Read the model definition and answer for the solid it produces. Units are mm, in the model's axes. A direction names the side the tool comes from. Coordinates: 2 decimals unless noted, no trailing zeros. Loops run counter-clockwise (first coordinate to the right, second up) from the corner with the lowest first, then second, coordinate; pieces in that order, holes last. Notation, with made-up numbers: (-7.5, 28) - (24.5, 28) arc R15 cw to (24.5, 56) - close; hole circle Ø9 at (29.5, -18). An arc over 180 degrees is marked (long way). Use one line per item in the form item = value.
from build123d import *

# Parameters (mm, degrees)
BOX001_W               = 4
BOX001_H               = 19
BOX001_DEPTH           = 10
BOX001_PLACEMENT_ANGLE = 90
POCKET001_DEPTH        = 5
BOX002_W               = 4
BOX002_H               = 19
BOX002_DEPTH           = 10
POCKET002_DEPTH        = 5
BOX003_W               = 4
BOX003_H               = 19
BOX003_DEPTH           = 10
BOX003_PLACEMENT_ANGLE = -90
POCKET003_DEPTH        = 5
BOX_W                  = 4
BOX_H                  = 19
BOX_DEPTH              = 10
POCKET_DEPTH           = 5
CYLINDER_R             = 3.5
CYLINDER_DEPTH         = 9
CYLINDER001_R          = 5
CYLINDER001_DEPTH      = 12


with BuildPart() as pocket001:
    # Box001 → Box001 (new body)
    with BuildSketch(Plane.XY):
        with Locations((2, 9.5)):
            Rectangle(BOX001_W, BOX001_H)
    extrude(amount=BOX001_DEPTH)


with BuildPart() as pocket001_1:
    # Box001 placement: moved
    add(pocket001.part.moved(Location((-4, -2, 0))).rotate(Axis((-4, -2, 0), (0, 0, 1)), BOX001_PLACEMENT_ANGLE))

    # Sketch001 → Pocket001 (cut)
    with BuildSketch(Plane(origin=(-4, 2, 0), x_dir=(-1, 0, 0), z_dir=(0, 1, 0))):
        Polygon((14.366066, 0), (19, 0), (19, 10), (17.795696, 10), align=None)
    extrude(amount=-POCKET001_DEPTH, mode=Mode.SUBTRACT)


with BuildPart() as pocket002:
    # Box002 → Box002 (new body)
    with BuildSketch(Plane(origin=(2, -4, 0), x_dir=(-1, 0, 0), z_dir=(0, 0, 1))):
        with Locations((2, 9.5)):
            Rectangle(BOX002_W, BOX002_H)
    extrude(amount=BOX002_DEPTH)

    # Sketch002 → Pocket002 (cut)
    with BuildSketch(Plane(origin=(-2, -4, 0), x_dir=(0, -1, 0), z_dir=(-1, 0, 0))):
        Polygon((14.366066, 0), (19, 0), (19, 10), (17.795696, 10), align=None)
    extrude(amount=-POCKET002_DEPTH, mode=Mode.SUBTRACT)


with BuildPart() as pocket003:
    # Box003 → Box003 (new body)
    with BuildSketch(Plane.XY):
        with Locations((2, 9.5)):
            Rectangle(BOX003_W, BOX003_H)
    extrude(amount=BOX003_DEPTH)


with BuildPart() as pocket003_1:
    # Box003 placement: moved
    add(pocket003.part.moved(Location((4, 2, 0))).rotate(Axis((4, 2, 0), (0, 0, 1)), BOX003_PLACEMENT_ANGLE))

    # Sketch003 → Pocket003 (cut)
    with BuildSketch(Plane(origin=(4, -2, 0), x_dir=(1, 0, 0), z_dir=(0, -1, 0))):
        Polygon((14.366066, 0), (19, 0), (19, 10), (17.795696, 10), align=None)
    extrude(amount=-POCKET003_DEPTH, mode=Mode.SUBTRACT)


with BuildPart() as fusion:
    # Box → Box (new body)
    with BuildSketch(Plane(origin=(-2, 4, 0), x_dir=(1, 0, 0), z_dir=(0, 0, 1))):
        with Locations((2, 9.5)):
            Rectangle(BOX_W, BOX_H)
    extrude(amount=BOX_DEPTH)

    # Sketch → Pocket (cut)
    with BuildSketch(Plane(origin=(2, 4, 0), x_dir=(0, 1, 0), z_dir=(1, 0, 0))):
        Polygon((14.366066, 0), (19, 0), (19, 10), (17.795696, 10), align=None)
    extrude(amount=-POCKET_DEPTH, mode=Mode.SUBTRACT)

    # Fusion: union Pocket001, Pocket002, Pocket003
    add(pocket001_1.part)
    add(pocket002.part)
    add(pocket003_1.part)


with BuildPart() as soporte:
    # Cone002 → Cone002 (revolve)
    with BuildSketch(Plane(origin=(0, 0, 10), x_dir=(1, 0, 0), z_dir=(0, -1, 0))):
        Polygon((0, 0), (5, 0), (25, 17), (0, 17), align=None)
    revolve(axis=Axis((0, 0, 10), (0, 0, 1)))


with BuildPart() as cilindro:
    # Cylinder → Cylinder (new body)
    with BuildSketch(Plane.XY):
        Circle(CYLINDER_R)
    extrude(amount=CYLINDER_DEPTH)


with BuildPart() as fusion001:
    # Cylinder001 → Cylinder001 (new body)
    with BuildSketch(Plane.XY):
        Circle(CYLINDER001_R)
    extrude(amount=CYLINDER001_DEPTH)

    # Cut001: cut Cilindro
    add(cilindro.part, mode=Mode.SUBTRACT)

    # Fusion001: union Fusion, Soporte
    add(fusion.part)
    add(soporte.part)


with BuildPart() as cono001:
    # Cone001 → Cone001 (revolve)
    with BuildSketch(Plane.XZ):
        Polygon((0, 0), (17, 0), (27, 27), (0, 27), align=None)
    revolve(axis=Axis((0, 0, 0), (0, 0, 1)))


with BuildPart() as obj1:
    # Cone → Cone (revolve)
    with BuildSketch(Plane.XZ):
        Polygon((0, 0), (20, 0), (30, 30), (0, 30), align=None)
    revolve(axis=Axis((0, 0, 0), (0, 0, 1)))

    # Cut: cut Cono001
    add(cono001.part, mode=Mode.SUBTRACT)

    # Fusion002: union Fusion001
    add(fusion001.part)


solid = obj1.part
Item 1: Find the intervals of material crossed by L1, parallel to X at y = 9, z = 15; L2, parallel to X at y = 5, z = 1; L3, parallel to Y at x = -7.5, z = 24.5, in increasing order.
Results below:
L1 = -23.32 to -20.68, -6.12 to 6.12, 20.68 to 23.32
L2 = -19.71 to -16.64, -2 to 2, 16.64 to 19.71
L3 = -27.15 to -24.97, -20.74 to 20.74, 24.97 to 27.15
Item 2: The part is cut by section A-A on x = 0. Give the vertices of the cut face in (y, z).
Results below:
outline = (-30, 30) - (-20, 0) - (-3.5, 0) - (-3.5, 9) - (3.5, 9) - (3.5, 0) - (20, 0) - (30, 30) - close; hole (-27, 27) - (-20.7, 10) - (-5, 10) - (-25, 27) - close; hole (5, 10) - (20.7, 10) - (27, 27) - (25, 27) - close
Item 3: The part is cut by section C-C on z = 21. Give the vertices of the cut face in (x, y), plus the area to 3 significant figures.
Results below:
outline = circle Ø54 at (0, 0); circle Ø35.88 at (0, 0); hole circle Ø49.56 at (0, 0)
area = 1,370 mm²
Item 4: The part is cut by section D-D on z = 5. Give the vertices of the cut face in (x, y).
Results below:
outline = circle Ø43.33 at (0, 0); hole (-18.75, -2) arc R18.85 ccw to (-2, -18.75) - (-2, -4.58) arc R5 cw to (-4.58, -2) - close; hole (-18.75, 2) - (-4.58, 2) arc R5 cw to (-2, 4.58) - (-2, 18.75) arc R18.85 ccw to start; hole circle Ø7 at (0, 0); hole (2, -18.75) arc R18.85 ccw to (18.75, -2) - (4.58, -2) arc R5 cw to (2, -4.58) - close; hole (2, 4.58) arc R5 cw to (4.58, 2) - (18.75, 2) arc R18.85 ccw to (2, 18.75) - close
Item 5: Each of these flat-tipped pins is pushed along its axis until it touches: P1, Ø8, axis at y = 12, z = 3, coming from the +X side; P2, Ø6, axis at x = -5, z = 25.5, coming from the +Y side; P3, Ø5, axis at y = 6, z = 13, coming from the -X side. Where does it stop, or does it pass through?
Results below:
P1 = 19.95
P2 = 29.17
P3 = -24.6
Item 6: Which of the six approach directions +Z, -Z, +X, -X, +Y, -Y give full straight-line access (tool end or side, diameter ignored) to faces 4 (the flat face through (-12, -2, 5)), 5 (the cylindrical face through (-3.52, 3.55, 4.93)), 6 (the flat face through (0, -4, 0))?
Results below:
face_4 = none
face_5 = -Z
face_6 = -Z, +X, -X, +Y, -Y
Item 7: For a pull along Y with two mould halves and no side action, classify faces 1 (the conical face through (10.54, -20.27, 8.54)), 2 (the flat face through (0, 0, 30)), 3 (the flat face through (12, 2, 5)) as +Y half, -Y half, draft (parallel to the pull), parting line (faces both ways), or undercut.
Results below:
face_1 = parting line
face_2 = draft
face_3 = undercut
